from build123d import *

# Parameters (mm, degrees)
SKETCH016_W   = 9
SKETCH016_H   = 23
PAD005_DEPTH  = 4.5
SKETCH018_R   = 1.6
SKETCH018_R_2 = 2.5
PAD006_DEPTH  = 4.5
PAD011_DEPTH  = 1.5


with BuildPart() as part:
    # Sketch016 → Pad005 (new body)
    with BuildSketch(Plane.XZ):
        with Locations((3, 11.5)):
            Rectangle(SKETCH016_W, SKETCH016_H)
        with BuildLine():
            ThreePointArc((4.75, 18), (3, 19.75), (1.25, 18))
            Line((1.25, 18), (1.25, 16))
            ThreePointArc((1.25, 16), (3, 14.25), (4.75, 16))
            Line((4.75, 16), (4.75, 18))
        make_face(mode=Mode.SUBTRACT)
        with BuildLine():
            ThreePointArc((4.75, 10), (3, 11.75), (1.25, 10))
            Line((1.25, 10), (1.25, 8))
            ThreePointArc((1.25, 8), (3, 6.25), (4.75, 8))
            Line((4.75, 8), (4.75, 10))
        make_face(mode=Mode.SUBTRACT)
    extrude(amount=PAD005_DEPTH)

    # Sketch018 → Pad006 (join)
    with BuildSketch(Plane.XY):
        with BuildLine():
            ThreePointArc((-3.8635384963, -28.0358910598), (0, -31), (3.8635384963, -28.0358910598))
            Line((3.8635384963, -28.0358910598), (7.5, -25.9363790317))
            Line((7.5, -25.9363790317), (7.5, -4.5))
            Line((7.5, -4.5), (7.5, 0))
            Line((-1.5, 0), (7.5, 0))
            Line((-1.5, 0), (-1.5, -4.5))
            Line((-1.5, -4.5), (-1.5, -5.2919007565))
            ThreePointArc((-1.5, -5.2919007565), (-2.9961743014, -6.3499170663), (-3.8635384963, -7.9641089402))
            Line((-5.75, -15), (-3.8635384963, -7.9641089402))
            Line((-5.75, -21), (-5.75, -15))
            Line((-3.8635384963, -28.0358910598), (-5.75, -21))
        make_face()
        with Locations((0, -27)):
            Circle(SKETCH018_R, mode=Mode.SUBTRACT)
        with Locations((0, -9)):
            Circle(SKETCH018_R, mode=Mode.SUBTRACT)
        with Locations((0, -18)):
            Circle(SKETCH018_R_2, mode=Mode.SUBTRACT)
    extrude(amount=PAD006_DEPTH)

    # Sketch034 (on DatumPlane) → Pad011 (join, symmetric)
    with BuildSketch(Plane.YZ.offset(7.5)):
        Polygon((-4.5, 23), (-25.5, 4.5), (-25.5, 0), (0, 0), (0, 23), align=None)
    extrude(amount=PAD011_DEPTH, both=True)


with BuildPart() as part_1:
    # Body002 placement: moved
    add(part.part.moved(Location((-30.5, -6, 8))))


solid = part_1.part
Design review of the part built by this model. Coordinates are the model's own, in mm. A direction names the side the tool comes from. Coordinates: 2 decimals unless noted, no trailing zeros. Write each loop counter-clockwise with the first axis right and the second up, starting at its lowest first coordinate (ties: lowest second). Pieces come first, ordered by that corner, then holes. Notation, with made-up numbers: (43, 89.5) - (63, 89.5) arc R30 ccw to (63, 112.5) - close; hole circle Ø6 at (87.25, 5.25). An arc over 180 degrees is marked (long way). One line per item, written item: value.
1) Insertion check: pin 1 (1 mm diameter, centred on x = -26.5, y = -18.5, fed in from +Z); pin 2 (4 mm diameter, centred on y = -7.5, z = 16, fed in from -X); pin 3 (1.9 mm diameter, centred on x = -30.5, y = -15, fed in from -Z); pin 4 (8 mm diameter, centred on x = -27.5, z = 22, fed in from -Y). Each pin has a flat end and moves straight along its axis. Give the tip position at first contact, or say it passes through.
Answer sheet:
pin 1: stops at z = 12.5
pin 2: stops at x = -32
pin 3: passes through
pin 4: stops at y = -23.72
2) For faces 4 (the face through (-30.6, -37, 10.2)), 5 (the face through (-27.46, -8.22, 27.75)), 6 (the face through (-28, -10.5, 22)), 7 (the face through (-22, -31.5, 10)), list the 3-axis set-ups (+Z, -Z, +X, -X, +Y, -Y) from which the entire face can be reached by the end or side of a thin tool; tool diameter is ignored.
Answer sheet:
face 4: +Z, -Z, -Y
face 5: +Y, -Y
face 6: +Z, -X, -Y
face 7: +Z, -Z, +X, -Y
3) Add section B-B (y = -33). State the section outline as (x, z) points, plus the area to 3 significant figures.
Answer sheet:
outline: (-34.64, 8) - (-32.1, 8) - (-32.1, 12.5) - (-34.64, 12.5) - close; (-28.9, 8) - (-24.84, 8) - (-24.84, 12.5) - (-28.9, 12.5) - close
area: 29.7 mm2
4) Add section D-D (z = 13.5). State the section outline as (x, y) points.
Answer sheet:
outline: (-32, -10.5) - (-24.5, -10.5) - (-24.5, -30.36) - (-21.5, -30.36) - (-21.5, -6) - (-32, -6) - close
5) To check wall thickness, follow probe 1 along Y at (x, z) = (-30.5, 10.45); probe 2 along X at (y, z) = (-8.5, 25.25); probe 3 along Z at (x, y) = (-35.5, -25.5). State the ranges of each line that lie inside material, in increasing order.
Answer sheet:
probe 1: y = -37 to -34.6, -31.4 to -26.5, -21.5 to -16.6, -13.4 to -6
probe 2: x = -32 to -29.25, -25.75 to -21.5
probe 3: z = 8 to 12.5
6) Mouldability with a two-part tool opening along Z and no side actions: class faces 1 (the face through (-35.32, -17.53, 10.22)), 2 (the face through (-27.54, -8.22, 14.25)), 3 (the face through (-27, -8, 31)) as +Z half, -Z half, draft (parallel to the pull), parting line (faces both ways), or undercut.
Answer sheet:
face 1: draft
face 2: undercut
face 3: +Z half
7) Add section A-A (x = -30.5). State the section outline as (y, z) points, plus the area to 3 significant figures.
Answer sheet:
outline: (-37, 8) - (-34.6, 8) - (-34.6, 12.5) - (-37, 12.5) - close; (-31.4, 8) - (-26.5, 8) - (-26.5, 12.5) - (-31.4, 12.5) - close; (-21.5, 8) - (-16.6, 8) - (-16.6, 12.5) - (-21.5, 12.5) - close; (-13.4, 8) - (-6, 8) - (-6, 31) - (-10.5, 31) - (-10.5, 12.5) - (-13.4, 12.5) - close
area: 171 mm2
8) Add section C-C (x = -22.25). State the section outline as (y, z) points.
Answer sheet:
outline: (-31.5, 8) - (-6, 8) - (-6, 31) - (-10.5, 31) - (-31.5, 12.5) - close
